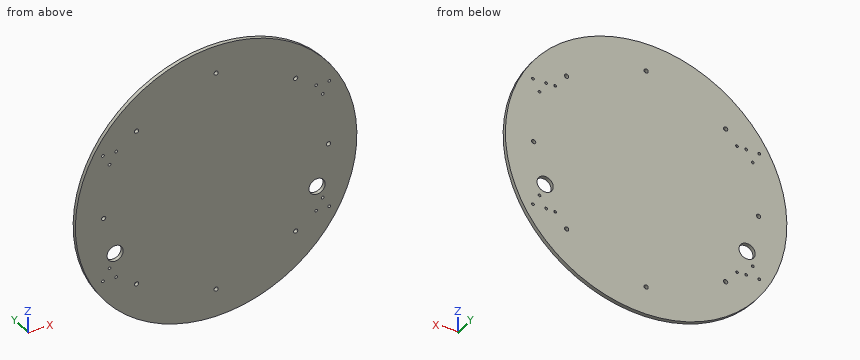
```python
from build123d import *

# Parameters (mm, degrees)
SKETCH1_R           = 177
BOSS_EXTRUDE1_DEPTH = 4.7625
SKETCH3_R           = 1.7
CUT_EXTRUDE1_DEPTH  = 2.54
SKETCH4_R           = 1.7
CUT_EXTRUDE2_DEPTH  = 251.361102023
SKETCH5_R           = 10.16
WIRES_2_DEPTH       = 251.361102023
SKETCH6_R           = 2.667
ZIP_TIES_DEPTH      = 251.361102023


with BuildPart() as part:
    # Sketch1 → Boss-Extrude1 (new body)
    with BuildSketch(Plane(origin=(0, 0, 0), x_dir=(1, 0, 0), z_dir=(0, 1, 0))):
        with Locations(Location((0, 0, 0), (0, 0, 90))):
            Circle(SKETCH1_R)
    extrude(amount=BOSS_EXTRUDE1_DEPTH)

    # Sketch3 → Cut-Extrude1 (cut)
    with BuildSketch(Plane(origin=(0, 4.7625, 0), x_dir=(1, 0, 0), z_dir=(0, 1, 0))):
        with Locations(Location((-114.3, -82.55, 0), (0, 0, 270))):
            Circle(SKETCH3_R)
        with Locations(Location((-114.3, 82.55, 0), (0, 0, 270))):
            Circle(SKETCH3_R)
        with Locations(Location((114.3, 82.55, 0), (0, 0, 270))):
            Circle(SKETCH3_R)
        with Locations(Location((114.3, -82.55, 0), (0, 0, 270))):
            Circle(SKETCH3_R)
    extrude(amount=-CUT_EXTRUDE1_DEPTH, mode=Mode.SUBTRACT)

    # Sketch4 → Cut-Extrude2 (cut, through all)
    with BuildSketch(Plane(origin=(0, 4.7625, 0), x_dir=(1, 0, 0), z_dir=(0, 1, 0))):
        with Locations(Location((142.287973842, -82.15, 0), (0, 0, 270))):
            Circle(SKETCH4_R)
        with Locations(Location((125.7901899, -82.15, 0), (0, 0, 270))):
            Circle(SKETCH4_R)
        with Locations(Location((134.039081871, -67.8625, 0), (0, 0, 270))):
            Circle(SKETCH4_R)
        with Locations(Location((-134.039081871, -67.8625, 0), (0, 0, 270))):
            Circle(SKETCH4_R)
        with Locations(Location((-125.7901899, -82.15, 0), (0, 0, 270))):
            Circle(SKETCH4_R)
        with Locations(Location((-142.287973842, -82.15, 0), (0, 0, 270))):
            Circle(SKETCH4_R)
        with Locations(Location((-142.287973842, 82.15, 0), (0, 0, 270))):
            Circle(SKETCH4_R)
        with Locations(Location((-125.7901899, 82.15, 0), (0, 0, 270))):
            Circle(SKETCH4_R)
        with Locations(Location((-134.039081871, 67.8625, 0), (0, 0, 270))):
            Circle(SKETCH4_R)
        with Locations(Location((134.039081871, 67.8625, 0), (0, 0, 270))):
            Circle(SKETCH4_R)
        with Locations(Location((125.7901899, 82.15, 0), (0, 0, 270))):
            Circle(SKETCH4_R)
        with Locations(Location((142.287973842, 82.15, 0), (0, 0, 270))):
            Circle(SKETCH4_R)
    extrude(amount=-CUT_EXTRUDE2_DEPTH, mode=Mode.SUBTRACT)

    # Sketch5 → Wires 2 (cut, through all)
    with BuildSketch(Plane(origin=(0, 4.7625, 0), x_dir=(1, 0, 0), z_dir=(0, 1, 0))):
        with Locations(Location((-127, 50.8, 0), (0, 0, 270))):
            Circle(SKETCH5_R)
        with Locations(Location((127, 50.8, 0), (0, 0, 270))):
            Circle(SKETCH5_R)
    extrude(amount=-WIRES_2_DEPTH, mode=Mode.SUBTRACT)

    # Sketch6 → Zip Ties (cut, through all)
    with BuildSketch(Plane(origin=(0, 4.7625, 0), x_dir=(1, 0, 0), z_dir=(0, 1, 0))):
        with Locations(Location((0, -141.44, 0), (0, 0, 270))):
            Circle(SKETCH6_R)
        with Locations(Location((-100.013183131, -100.013183131, 0), (0, 0, 270))):
            Circle(SKETCH6_R)
        with Locations(Location((-141.44, 0, 0), (0, 0, 270))):
            Circle(SKETCH6_R)
        with Locations(Location((-100.013183131, 100.013183131, 0), (0, 0, 270))):
            Circle(SKETCH6_R)
        with Locations(Location((0, 141.44, 0), (0, 0, 270))):
            Circle(SKETCH6_R)
        with Locations(Location((100.013183131, 100.013183131, 0), (0, 0, 270))):
            Circle(SKETCH6_R)
        with Locations(Location((141.44, 0, 0), (0, 0, 270))):
            Circle(SKETCH6_R)
        with Locations(Location((100.013183131, -100.013183131, 0), (0, 0, 270))):
            Circle(SKETCH6_R)
    extrude(amount=-ZIP_TIES_DEPTH, mode=Mode.SUBTRACT)


solid = part.part
```
Verification items for the finished model (mm, model axes). Coordinates: 2 decimals unless noted, no trailing zeros. Order: outer loops, then holes, each group sorted by start corner. A loop starts at its lowest first (then second) coordinate and runs counter-clockwise, first axis right, second up. Notation, with made-up numbers: (37, 44) -> (71, 44) arc R15 cw to (71, 67) -> close; hole circle Ø2 at (4, 28.25). An arc over 180 degrees is marked (long way). Put each result on its own line as item: value. Start each with the question number.
1) Cross-section at B-B (x = -49.5). Enter the section's corners in (y, z).
2) Material ranges on L1, parallel to X at y = 1.7, z = -82.15; L2, parallel to X at y = 2.95, z = 0; L3, parallel to Z at x = -125, y = 4.4, recorded low to high.
3) Go/stop test with flat-tipped pins: pin 1 (2.5 mm diameter, centred on x = -125.79, z = 82.15, fed in from +Y); pin 2 (1 mm diameter, centred on x = 131, y = 3.5, fed in from -Z); pin 3 (2 mm diameter, centred on x = -114.3, z = 82.55, fed in from +Y); pin 4 (1 mm diameter, centred on x = 102.5, y = 3, fed in from +Z). Record where each tip stops, or that it passes through.
4) Cross-section at C-C (z = 39.5). Enter the section's corners in (x, y), plus the area to 3 significant figures.
5) Cross-section at A-A (y = 4). State how many separate pieces and enclosed holes the cut face has, plus the area to 3 significant figures.
Geometry check:
1. outline: (0, -169.94) -> (4.76, -169.94) -> (4.76, 169.94) -> (0, 169.94) -> close
2. L1: x = -156.78 to -143.99, -140.59 to -127.49, -124.09 to 124.09, 127.49 to 140.59, 143.99 to 156.78
2. L2: x = -177 to -144.11, -138.77 to 138.77, 144.11 to 177
2. L3: z = -125.32 to -83.66, -80.64 to -60.76, -40.84 to 80.64, 83.66 to 125.32
3. pin 1: passes through
3. pin 2: stops at z = -119.58
3. pin 3: stops at y = 2.22
3. pin 4: stops at z = 144.65
4. outline: (-172.54, 0) -> (172.54, 0) -> (172.54, 4.76) -> (-172.54, 4.76) -> close
4. area: 1,640 mm^2
5. separate pieces: 1
5. enclosed holes: 26
5. area: 97,500 mm^2
